Could you check a few things on this model? Use its own coordinates, in mm. Face numbers are marked on the shaded views. A direction names the side the tool comes from. Coordinates: 2 decimals unless noted, no trailing zeros. Order: outer loops, then holes, each group sorted by start corner. A loop starts at its lowest first (then second) coordinate and runs counter-clockwise, first axis right, second up. Notation, with made-up numbers: (61, 53) -> (99, 53) arc R18 cw to (99, 84) -> close; hole circle Ø4 at (-3.5, 10.5). An arc over 180 degrees is marked (long way). Use a Markdown table: item, result. Add a question column.
1) If we section it at A-A (z = 22): Write out the boundary of the cut face in (x, y).
2) Will these pins go through, and if not, where does the flat tip stop? pin 1 Ø8 at (x, y) = (-27.5, 28) entering from -Z; pin 2 Ø8 at (y, z) = (0, 64) entering from +X; pin 3 Ø1 at (x, y) = (26, -42.5) entering from +Z.
3) Which directions (+Z, -Z, +X, -X, +Y, -Y) give clear straight access to the entire face, cutting with the end or side of a thin tool? Please do the marked faces 1 and 2.
4) If we section it at B-B (z = 82.5): Write out the boundary of the cut face in (x, y) (3 decimals), plus the area to 3 significant figures.
5) Thinking about a two-plate mould opening in Z: for the marked faces 3, 4 and 5, which applies, +Z half, -Z half, draft (parallel to the pull), parting line (faces both ways), or undercut?
6) If I drill on L1, parallel to X at y = -21, z = 64.5; L2, parallel to X at y = -10, z = 76; L3, parallel to Y at x = 3, z = 61.5, over which ranges is the centre line in solid material (lowest first)? Write a range as [from, to].
Autodesk Fusion 360 part; units mm, degrees
sketch "Sketch1" plane through (0, 0, 0) normal (0, 0, 1) x (1, 0, 0)
  circle A0 centre (0, 0) radius 50
  circle A1 centre (0, 0) radius 47
  dimension "d1" = 100
  dimension "d9" = -3
ref_plane "WorkPlane1" through (0, 0, 41) normal (0, 0, 1) x (1, 0, 0)
sketch "Sketch2" plane through (0, 0, 41) normal (0, 0, 1) x (1, 0, 0)
  circle A0 centre (0, 0) radius 51
  circle A1 centre (0, 0) radius 48
  dimension "d4" = 102
  dimension "d10" = -3
ref_plane "WorkPlane2" through (0, 0, 66) normal (0, 0, 1) x (1, 0, 0)
sketch "Sketch5" plane through (0, 0, 66) normal (0, 0, 1) x (1, 0, 0)
  circle A0 centre (0, 0) radius 29.75
  circle A1 centre (0, 0) radius 27.75
  dimension "d22" = 59.5
  dimension "d23" = -2
ref_plane "WorkPlane3" through (0, 0, 91) normal (0, 0, 1) x (1, 0, 0)
sketch "Sketch6" plane through (0, 0, 91) normal (0, 0, 1) x (1, 0, 0)
  circle A0 centre (0, 0) radius 29
  circle A1 centre (0, 0) radius 27
  dimension "d25" = 58
  dimension "d26" = -2
sketch "Sketch7" plane through (0, 0, 0) normal (0, 1, 0) x (1, 0, 0)
  line L0 (-47, 0) -> (47, 0)
  line L1 (-50, 0) -> (50, 0)
  line L2 (-51, -41) -> (51, -41)
  line L3 (-48, -41) -> (48, -41)
  line L4 (-27.75, -66) -> (27.75, -66)
  line L5 (-29.75, -66) -> (29.75, -66)
  line L6 (-27, -91) -> (27, -91)
  line L7 (-29, -91) -> (29, -91)
  line L8 (-50, 0) -> (-51, -41)
  line L9 (-47, 0) -> (-48, -41)
  line L10 (-48, -41) -> (-27.75, -66)
  line L11 (-51, -41) -> (-29.75, -66)
  line L12 (-29.75, -66) -> (-29, -91)
  line L13 (-27.75, -66) -> (-27, -91)
  line L14 (-51, -41) -> (-56, -41)
  line L15 (-56, -41) -> (-56, -36)
  line L16 (-56, -36) -> (-51, -36)
  line L17 (-51, -36) -> (-51, -41) construction
  line L18 (-51, -36) -> (-50.878, -36)
  line L19 (0, 0) -> (0, -91) construction
  dimension "d27" = 5
  dimension "d28" = 5
revolve "Revolve2" add sketch "Sketch7" angle 360 about axis through (0, 0, 0) along (0, 0, 1)
fillet "Fillet4" radius 40 1 edges at (-44.7517, 17.3575, 41)
fillet "Fillet5" radius 25 1 edges at (-25.8721, 10.0348, 66)
fillet "Fillet6" radius 20 1 edges at (-27.7367, 10.7581, 66)
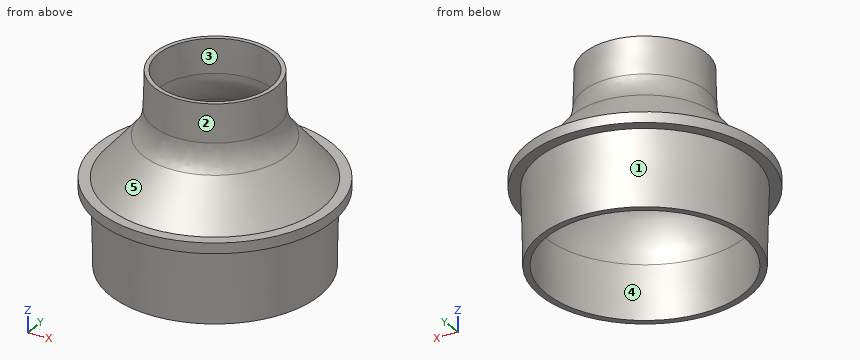
Answer sheet:
| question | item | result |
|---|---|---|
| 1 | outline | circle Ø101.07 at (0, 0); hole circle Ø95.07 at (0, 0) |
| 2 | pin 1 | z = 45.51 |
| 2 | pin 2 | x = 34.85 |
| 2 | pin 3 | z = 42.97 |
| 3 | face 1 | -Z |
| 3 | face 2 | +Z |
| 4 | outline | circle Ø58.51 at (0, 0); hole circle Ø54.51 at (0, 0) |
| 4 | area | 355 mm2 |
| 5 | face 3 | -Z half |
| 5 | face 4 | undercut |
| 5 | face 5 | +Z half |
| 6 | L1 | [-23.78, -21.26], [21.26, 23.78] |
| 6 | L2 | [-27.7, -25.56], [25.56, 27.7] |
| 6 | L3 | [-33.48, -31.42], [31.42, 33.48] |
